Input: part model. Units: mm. Frame: model coordinates. Coordinates: 2 decimals unless noted, no trailing zeros. Write each loop counter-clockwise with the first axis right and the second up, starting at its lowest first coordinate (ties: lowest second). Pieces come first, ordered by that corner, then holes. Notation, with made-up numbers: (57.25, -1) -> (74.25, -1) arc R10 cw to (74.25, 4) -> close; hole circle Ø1 at (36, 69.5). An arc over 180 degrees is marked (long way). Use one line per item in the form item = value. Start each with the question number.
(1) Cut plane A-A on x = 31.3. Return the cut outline in (y, z), plus the area to 3 significant figures.
(2) Cut plane C-C on y = 1.7. State how many separate pieces and enclosed holes the cut face has, plus the area to 3 significant figures.
(3) Cut plane D-D on x = 81.3. Return the cut outline in (y, z).
(4) First-contact query: pin 1 (1.5 mm diameter, centred on y = 1.5, z = 15.5, fed in from -X); pin 2 (0.9 mm diameter, centred on x = -22.5, y = 2, fed in from +Z); pin 3 (1.5 mm diameter, centred on x = -22.5, y = 2, fed in from -Z); pin 4 (1.8 mm diameter, centred on x = 81.3, z = 0, fed in from +Y). Flat tips, straight axial feed; report the tip coordinate or a pass-through.
(5) Ray query, line 1 along Z through (x, y) = (-22.8, 1.7); line 2 along Z through (x, y) = (14.3, 1.5); line 3 along Z through (x, y) = (102.5, 2.4). Return the intervals inside material, ascending.
(6) Cut plane B-B on x = -22.8. Return the cut outline in (y, z).
```python
from build123d import *

# Parameters (mm, degrees)
ESBO_O1_R                = 1.5
ESBO_O1_W                = 3
ESBO_O1_H                = 8
ESBO_O1_W_2              = 8
ESBO_O1_H_2              = 3
RESSALTO_EXTRUS_O1_DEPTH = 3


with BuildPart() as part:
    # Esboço1 → Ressalto-extrusão1 (new body)
    with BuildSketch(Plane(origin=(0, 0, 0), x_dir=(1, 0, 0), z_dir=(0, 1, 0))):
        with BuildLine():
            ThreePointArc((-19.544028008, 21.987058404), (-23.767751262, 20.202130438), (-26.75078073, 16.719697214))
            ThreePointArc((-26.75078073, 16.719697214), (-30.815641586, -2.3e-07), (-26.750780519, -16.719697622))
            ThreePointArc((-26.750780519, -16.719697622), (-23.767751269, -20.202130616), (-19.544028371, -21.987058612))
            add(Edge.make_bspline(
                [(23.247280819, -14.466941833), (22.21541658, -14.85491506), (7.843575487, -20.128766531), (-8.032505645, -23.945383183), (-19.544028371, -21.987058612)],
                knots=[0.1894974, 0.1894974, 0.1894974, 0.1894974, 0.216439611, 0.561126756, 0.561126756, 0.561126756, 0.561126756], degree=3))
            ThreePointArc((23.247280819, -14.466941833), (53.114593998, -6.632399806), (83.953283265, -5.079438247))
            add(Edge.make_bspline(
                [(97.598521861, -6.15), (93.039003458, -5.676054912), (88.490590593, -5.319200994), (83.953283265, -5.079438247)],
                knots=[0, 0, 0, 0, 0.137959586, 0.137959586, 0.137959586, 0.137959586], degree=3))
            add(Edge.make_bspline(
                [(114.569723425, -4.259468977), (109.134912936, -6.157348784), (103.477845748, -6.787525792), (97.598521861, -6.15)],
                knots=[0.35388944, 0.35388944, 0.35388944, 0.35388944, 1, 1, 1, 1], degree=3))
            ThreePointArc((114.569723425, -4.259468977), (117.037611185, -3.468795912), (119.543150354, -2.807050219))
            add(Edge.make_bspline(
                [(119.543150354, -2.807050219), (131.408766059, 0), (119.543150354, 2.807050219)],
                knots=[5.194112445, 5.194112445, 5.194112445, 7.372258169, 7.372258169, 7.372258169], degree=2, weights=[1, 0.463307193, 1]))
            ThreePointArc((119.543150354, 2.807050219), (117.037611185, 3.468795912), (114.569723425, 4.259468977))
            add(Edge.make_bspline(
                [(114.569723425, 4.259468977), (109.134912936, 6.157348784), (103.477845748, 6.787525792), (97.598521861, 6.15)],
                knots=[0.35388944, 0.35388944, 0.35388944, 0.35388944, 1, 1, 1, 1], degree=3))
            add(Edge.make_bspline(
                [(97.598521861, 6.15), (93.039003574, 5.676054924), (88.490590825, 5.319201013), (83.953283612, 5.079438265)],
                knots=[0, 0, 0, 0, 0.137959582, 0.137959582, 0.137959582, 0.137959582], degree=3))
            ThreePointArc((83.953283612, 5.079438265), (53.114594943, 6.632399691), (23.24728229, 14.466941345))
            add(Edge.make_bspline(
                [(23.24728229, 14.466941345), (22.21541757, 14.854914742), (7.843576153, 20.128766099), (-8.032505406, 23.945382333), (-19.544028008, 21.987058404)],
                knots=[0.189497388, 0.189497388, 0.189497388, 0.189497388, 0.216439611, 0.561126752, 0.561126752, 0.561126752, 0.561126752], degree=3))
        make_face()
        with Locations((-22.8, -14.3)):
            Circle(ESBO_O1_R, mode=Mode.SUBTRACT)
        with Locations((0.2, -14.3)):
            Rectangle(ESBO_O1_W, ESBO_O1_H, mode=Mode.SUBTRACT)
        with Locations((-14.3, -11.5)):
            Rectangle(ESBO_O1_W_2, ESBO_O1_H_2, mode=Mode.SUBTRACT)
        with Locations((14.3, -11.5)):
            Circle(ESBO_O1_R, mode=Mode.SUBTRACT)
        with Locations((-6.3, 0)):
            Circle(ESBO_O1_R, mode=Mode.SUBTRACT)
        with Locations((6.3, 0)):
            Circle(ESBO_O1_R, mode=Mode.SUBTRACT)
        with Locations((-14.3, 11.5)):
            Circle(ESBO_O1_R, mode=Mode.SUBTRACT)
        with Locations((31.3, 0)):
            Circle(ESBO_O1_R, mode=Mode.SUBTRACT)
        with Locations((14.3, 11.500000009)):
            Rectangle(ESBO_O1_W_2, ESBO_O1_H_2, mode=Mode.SUBTRACT)
        with Locations((-22.8, 14.3)):
            Rectangle(ESBO_O1_W, ESBO_O1_H, mode=Mode.SUBTRACT)
        with Locations((0.2, 14.3)):
            Circle(ESBO_O1_R, mode=Mode.SUBTRACT)
        Polygon((60.3, -1.5), (56.3, -1.5), (52.3, -1.5), (52.3, 1.5), (60.3, 1.5), align=None, mode=Mode.SUBTRACT)
        with Locations((81.3, 0)):
            Circle(ESBO_O1_R, mode=Mode.SUBTRACT)
        with Locations((106.3, 0)):
            Circle(ESBO_O1_R, mode=Mode.SUBTRACT)
    extrude(amount=RESSALTO_EXTRUS_O1_DEPTH)


solid = part.part
```
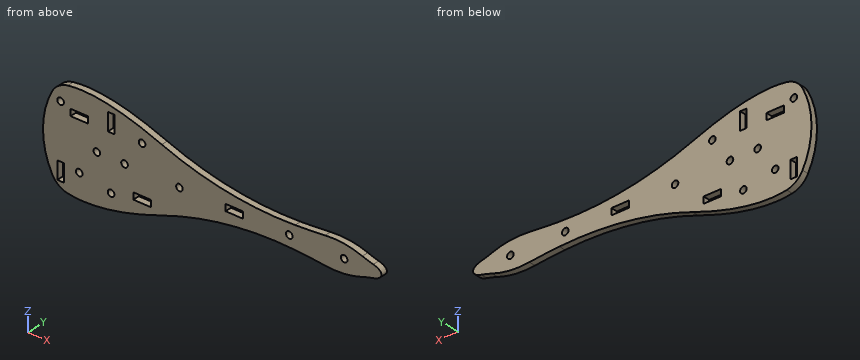
Values:
q1.outline = (0, -11.7) -> (3, -11.7) -> (3, -1.5) -> (0, -1.5) -> close; (0, 1.5) -> (3, 1.5) -> (3, 11.7) -> (0, 11.7) -> close
q1.area = 61.2 mm2
q2.separate_pieces = 1
q2.enclosed_holes = 14
q2.area = 3,240 mm2
q3.outline = (0, -4.96) -> (3, -4.96) -> (3, -1.5) -> (0, -1.5) -> close; (0, 1.5) -> (3, 1.5) -> (3, 4.96) -> (0, 4.96) -> close
q4.pin_1 = -27.69
q4.pin_2 = 21.21
q4.pin_3 = -21.34
q4.pin_4 = through
q5.line_1 = -20.83 to -18.3, -10.3 to 12.8, 15.8 to 20.83
q5.line_2 = -17.58 to -13, -10 to 10, 13 to 17.58
q5.line_3 = -6.39 to 6.39
q6.outline = (0, -20.83) -> (3, -20.83) -> (3, -18.3) -> (0, -18.3) -> close; (0, -10.3) -> (3, -10.3) -> (3, 12.8) -> (0, 12.8) -> close; (0, 15.8) -> (3, 15.8) -> (3, 20.83) -> (0, 20.83) -> close
